Build history of the part. All positions in model axes, mm. A direction names the side the tool comes from. Coordinates: 2 decimals unless noted, no trailing zeros. Order: outer loops, then holes, each group sorted by start corner. A loop starts at its lowest first (then second) coordinate and runs counter-clockwise, first axis right, second up. Notation, with made-up numbers: (80, -6) -> (119, -6) arc R11 ccw to (119, 7) -> close; hole circle Ø10 at (52, 0). An arc over 180 degrees is marked (long way). Write each question's results on one line, items separated by ' | '.
from build123d import *

# Parameters (mm, degrees)
CROQUIS1_W              = 150
CROQUIS1_H              = 50.8
SALIENTE_EXTRUIR1_DEPTH = 20
CROQUIS2_R              = 2.75
CORTAR_EXTRUIR1_DEPTH   = 21
CROQUIS3_R              = 5
CORTAR_EXTRUIR2_DEPTH   = 5
CHAFL_N1_SIZE           = 2
CHAFL_N2_SIZE           = 2
CHAFL_N3_SIZE           = 2


with BuildPart() as part:
    # Croquis1 → Saliente-Extruir1 (new body)
    with BuildSketch(Plane.XY):
        Rectangle(CROQUIS1_W, CROQUIS1_H)
    extrude(amount=SALIENTE_EXTRUIR1_DEPTH)

    # Croquis2 → Cortar-Extruir1 (cut, through all)
    with BuildSketch(Plane(origin=(0, 0, 0), x_dir=(-1, 0, 0), z_dir=(0, 0, -1))):
        with Locations((0, 9.55)):
            Circle(CROQUIS2_R)
        with Locations((0, -9.55)):
            Circle(CROQUIS2_R)
        with Locations((30, 0)):
            Circle(CROQUIS2_R)
        with Locations((-30, 0)):
            Circle(CROQUIS2_R)
    extrude(amount=-CORTAR_EXTRUIR1_DEPTH, mode=Mode.SUBTRACT)

    # Croquis3 → Cortar-Extruir2 (cut)
    with BuildSketch(Plane(origin=(0, 0, 0), x_dir=(-1, 0, 0), z_dir=(0, 0, -1))):
        with Locations((0, 9.55)):
            Circle(CROQUIS3_R)
        with Locations((0, -9.55)):
            Circle(CROQUIS3_R)
    extrude(amount=-CORTAR_EXTRUIR2_DEPTH, mode=Mode.SUBTRACT)

    # Chaflán1
    chafl_n1_edges = [part.edges().sort_by_distance(p)[0] for p in [
        (0, -25.4, 0),
        (-75, 0, 0),
        (0, 25.4, 0),
        (75, 0, 0),
    ]]
    chamfer(chafl_n1_edges, length=CHAFL_N1_SIZE)

    # Chaflán2
    chafl_n2_edges = [part.edges().sort_by_distance(p)[0] for p in [
        (-75, 0, 20),
        (0, -25.4, 20),
        (75, 0, 20),
        (0, 25.4, 20),
    ]]
    chamfer(chafl_n2_edges, length=CHAFL_N2_SIZE)

    # Chaflán3
    chafl_n3_edges = [part.edges().sort_by_distance(p)[0] for p in [
        (-75, 25.4, 10),
        (-75, -25.4, 10),
        (75, 25.4, 10),
        (75, -25.4, 10),
    ]]
    chamfer(chafl_n3_edges, length=CHAFL_N3_SIZE)


solid = part.part
Item 1: Drill centre lines: line 1 (Y direction, x = 0, z = 2.55); line 2 (X direction, y = -9, z = 3.75); line 3 (Y direction, x = 0, z = 1.15). Where is each one in solid material? Low to high. Write a range as from..to.
Answer:
line 1: y = -25.4..-14.55, -4.55..4.55, 14.55..25.4 | line 2: x = -75..-4.97, 4.97..75 | line 3: y = -24.55..-14.55, -4.55..4.55, 14.55..24.55
Item 2: Pull direction Y, two halves, no side cores. Call faces 1 (the cylindrical face through (0.358, -6.823, 12.395)), 2 (the flat face through (-1, 0, 20)), 3 (the flat face through (-1, -25.4, 10)): released by +Y, released by -Y, zero draft, split by the parting line, or undercut.
Answer:
face 1: undercut | face 2: zero draft | face 3: released by -Y
Item 3: Slice it at B-B, the plane y = 9.55. List the corners of the cut face in (x, z), and give its area (3 significant figures).
Answer:
outline: (-75, 2) -> (-73, 0) -> (-5, 0) -> (-5, 5) -> (-2.75, 5) -> (-2.75, 20) -> (-73, 20) -> (-75, 18) -> close; (2.75, 5) -> (5, 5) -> (5, 0) -> (73, 0) -> (75, 2) -> (75, 18) -> (73, 20) -> (2.75, 20) -> close | area: 2,860 mm^2
Item 4: Slice it at A-A, the plane x = -30. List the corners of the cut face in (y, z), and give its area (3 significant figures).
Answer:
outline: (-25.4, 2) -> (-23.4, 0) -> (-2.75, 0) -> (-2.75, 20) -> (-23.4, 20) -> (-25.4, 18) -> close; (2.75, 0) -> (23.4, 0) -> (25.4, 2) -> (25.4, 18) -> (23.4, 20) -> (2.75, 20) -> close | area: 898 mm^2
Item 5: Slice it at C-C, the plane x = 0. List the corners of the cut face in (y, z).
Answer:
outline: (-25.4, 2) -> (-23.4, 0) -> (-14.55, 0) -> (-14.55, 5) -> (-12.3, 5) -> (-12.3, 20) -> (-23.4, 20) -> (-25.4, 18) -> close; (-6.8, 5) -> (-4.55, 5) -> (-4.55, 0) -> (4.55, 0) -> (4.55, 5) -> (6.8, 5) -> (6.8, 20) -> (-6.8, 20) -> close; (12.3, 5) -> (14.55, 5) -> (14.55, 0) -> (23.4, 0) -> (25.4, 2) -> (25.4, 18) -> (23.4, 20) -> (12.3, 20) -> close
Item 6: Pin check, flat tip, straight feed: pin 1 (7 mm diameter, centred on x = 0, y = -9.55, fed in from -Z). Stop position of the tip, or through.
Answer:
pin 1: stops at z = 5
Item 7: Tool access for faces 4 (the cylindrical face through (0.596, 6.865, 12.395)), 5 (the cylindrical face through (1.08, 4.67, 2.46)): list every direction of +Z, -Z, +X, -X, +Y, -Y with a clear straight run to the whole face (end or side of a thin tool).
Answer:
face 4: +Z, -Z | face 5: -Z
